```python
from build123d import *

# Parameters (mm, degrees)
PAD_DEPTH       = 7
SKETCH002_R     = 4.1
POCKET001_DEPTH = 10.5
SKETCH003_R     = 2.25
HOLE_DEPTH      = 7.001
POCKET002_DEPTH = 3.001


with BuildPart() as part:
    # Sketch001 → Pad (new body)
    with BuildSketch(Plane.XY):
        with BuildLine():
            ThreePointArc((-7, 21), (-17.606602, 16.606602), (-22, 6))
            Line((-22, 0), (-22, 6))
            ThreePointArc((-22, 0), (-17.606602, -10.606602), (-7, -15))
            Line((7, -15), (-7, -15))
            ThreePointArc((7, -15), (17.606602, -10.606602), (22, 0))
            Line((22, 6), (22, 0))
            ThreePointArc((22, 6), (17.606602, 16.606602), (7, 21))
            Line((-7, 21), (7, 21))
        make_face()
    extrude(amount=PAD_DEPTH)

    # Sketch002 → Pocket001 (cut, symmetric)
    with BuildSketch(Plane.XZ):
        with Locations((0, 5)):
            Circle(SKETCH002_R)
    extrude(amount=POCKET001_DEPTH, both=True, mode=Mode.SUBTRACT)

    # Sketch003 → Hole (cut, through all)
    with BuildSketch(Plane(origin=(12, 12, 0), x_dir=(1, 0, 0), z_dir=(0, 0, 1))):
        Circle(SKETCH003_R)
        with Locations((-24, 0)):
            Circle(SKETCH003_R)
    extrude(amount=HOLE_DEPTH, mode=Mode.SUBTRACT)

    # Sketch004 (on Sketch) → Pocket002 (cut, through all)
    with BuildSketch(Plane(origin=(12, 12, 4), x_dir=(1, 0, 0), z_dir=(0, 0, 1))):
        Polygon((4.214657, 0), (2.107328, 3.65), (-2.107328, 3.65), (-4.214657, 0), (-2.107328, -3.65), (2.107328, -3.65), align=None)
        Polygon((-19.785343, 0), (-21.892672, 3.65), (-26.107328, 3.65), (-28.214657, 0), (-26.107328, -3.65), (-21.892672, -3.65), align=None)
    extrude(amount=POCKET002_DEPTH, mode=Mode.SUBTRACT)

    # Sketch → Groove (revolve, cut)
    with BuildSketch(Plane.XY.offset(5)):
        with BuildLine():
            ThreePointArc((10.5, -6), (16.5, 0), (10.5, 6))
            Line((9, 6), (10.5, 6))
            Line((8, 5), (9, 6))
            Line((0, 5), (8, 5))
            Line((0, 5), (0, -5))
            Line((0, -5), (8, -5))
            Line((8, -5), (9, -6))
            Line((9, -6), (10.5, -6))
        make_face()
    revolve(axis=Axis((0, 0, 5), (0, 1, 0)), mode=Mode.SUBTRACT)


solid = part.part
```
Work out the finished part from the listing and answer in its coordinate system (mm). A direction names the side the tool comes from. Coordinates: 2 decimals unless noted, no trailing zeros. Write each loop counter-clockwise with the first axis right and the second up, starting at its lowest first coordinate (ties: lowest second). Pieces come first, ordered by that corner, then holes.
Q1. Determine the mould class of faces 1 (the face through (17.49, -10.72, 3.45)), 2 (the face through (0, -15, 3)), 3 (the face through (-8.824, 13.799, 5.479)), 4 (the face through (14, 14, 4)) for opening direction X: released by +X, released by -X, zero draft, split by the parting line, or undercut.
Q2. A cutting plane is placed at C-C, the plane z = 5. State how many separate pieces and enclosed holes the cut face has, then the cut area to 3 significant figures.
Q3. Each of these flat-tipped pins is pushed along its axis until it touches: pin 1 Ø1.5 at (x, z) = (11.5, 5.5) entering from -Y; pin 2 Ø2 at (x, y) = (11, 10.5) entering from +Z; pin 3 Ø1.5 at (x, z) = (-9, 4) entering from +Y. Where does it stop, or does it pass through?
Q4. A cutting plane is placed at A-A, the plane x = 0. Give the vertices of the cut face in (y, z), then the cut area to 3 significant figures.
Q5. A cutting plane is placed at D-D, the plane x = -5.5. Give the vertices of the cut face in (y, z), then the cut area to 3 significant figures.
Q6. A cutting plane is placed at B-B, the plane y = 2.5. Give the vertices of the cut face in (x, z).
Q7. Find the intervals of material crossed by line 1 (Y direction, x = -1.5, z = 3.75); line 2 (X direction, y = 12, z = 2.6); line 3 (X direction, y = 9, z = 6), in increasing order.
Q8. Which of the six approach directions +Z, -Z, +X, -X, +Y, -Y give full straight-line access (tool end or side, diameter ignored) to faces 5 (the face through (9, -6, 3)), 6 (the face through (15.176, 13.799, 5.479)), 7 (the face through (0, 21, 3))?
Findings below:
1. face 1: released by +X
1. face 2: zero draft
1. face 3: undercut
1. face 4: undercut
2. separate pieces: 1
2. enclosed holes: 3
2. area: 877 mm2
3. pin 1: stops at y = -14.52
3. pin 2: stops at z = 4
3. pin 3: stops at y = 20.95
4. outline: (-15, 0) - (-5, 0) - (-5, 0.9) - (-10.5, 0.9) - (-10.5, 7) - (-15, 7) - close; (5, 0) - (21, 0) - (21, 7) - (10.5, 7) - (10.5, 0.9) - (5, 0.9) - close
4. area: 115 mm2
5. outline: (-15, 0) - (-5, 0) - (-5, 7) - (-15, 7) - close; (5, 0) - (21, 0) - (21, 7) - (5, 7) - close
5. area: 182 mm2
6. outline: (-22, 0) - (-15.15, 0) arc R15.95 cw to (-15.83, 7) - (-22, 7) - close; (15.15, 0) - (22, 0) - (22, 7) - (15.83, 7) arc R15.95 cw to start
7. line 1: y = -15 to -10.5, 10.5 to 21
7. line 2: x = -20.75 to -14.25, -9.75 to 9.75, 14.25 to 20.75
7. line 3: x = -21.7 to -14.48, -9.52 to -3.98, 3.98 to 9.52, 14.48 to 21.7
8. face 5: none
8. face 6: +Z
8. face 7: +Z, -Z, +X, -X, +Y
